```python
from build123d import *

# Parameters (mm, degrees)
SKETCH_1_R          = 40
EXTRUDE_1_DEPTH     = 50
CUT_EXTRUDE_1_DEPTH = 30
CUT_EXTRUDE_2_DEPTH = 76.498344353


with BuildPart() as part:
    # Sketch 1 → Extrude 1 (new body)
    with BuildSketch(Plane(origin=(0, 0, 0), x_dir=(1, 0, 0), z_dir=(0, 1, 0))):
        with Locations(Location((0, 0, 0), (0, 0, 270))):
            Circle(SKETCH_1_R)
    extrude(amount=EXTRUDE_1_DEPTH)

    # Sketch 2 → Cut-Extrude 1 (cut)
    with BuildSketch(Plane.XZ):
        with BuildLine():
            Line((18.540496218, 7.5), (25, 7.5))
            Line((25, 7.5), (25, -7.5))
            Line((25, -7.5), (18.540496218, -7.5))
            ThreePointArc((18.540496218, -7.5), (-20, 0), (18.540496218, 7.5))
        make_face()
    extrude(amount=-CUT_EXTRUDE_1_DEPTH, mode=Mode.SUBTRACT)

    # Sketch 4 → Cut-Extrude 2 (cut, through all)
    with BuildSketch(Plane.XZ):
        with BuildLine():
            Line((40, -2.5), (30, -2.5))
            ThreePointArc((30, -2.5), (27.5, 0), (30, 2.5))
            Line((30, 2.5), (40, 2.5))
            ThreePointArc((40, 2.5), (42.5, 0), (40, -2.5))
        make_face()
    extrude(amount=-CUT_EXTRUDE_2_DEPTH, mode=Mode.SUBTRACT)


solid = part.part
```
The model under review builds one solid part; all positions refer to its coordinate system, in mm. A direction names the side the tool comes from. Round coordinates to 2 decimals unless told otherwise and drop trailing zeros. Write each loop counter-clockwise with the first axis right and the second up, starting at its lowest first coordinate (ties: lowest second). Pieces come first, ordered by that corner, then holes. Notation, with made-up numbers: (67.25, -9.75) -> (111.25, -9.75) arc R12 ccw to (111.25, -1.75) -> close; hole circle Ø7 at (5.5, 19.5). An arc over 180 degrees is marked (long way). Use CSV: the item, a comma, the result in double quotes.
Q1. Consider section A-A (y = 22.5). Give the boundary of the cut face in (x, z).
Checks:
outline,"(30, -2.5) arc R2.5 cw to (30, 2.5) -> (39.92, 2.5) arc R40 ccw (long way) to (39.92, -2.5) -> close; hole (18.54, -7.5) -> (25, -7.5) -> (25, 7.5) -> (18.54, 7.5) arc R20 ccw (long way) to start"
Q2. Consider section B-B (z = 0). Give the boundary of the cut face in (x, y), then the cut area to 4 significant figures.
Checks:
outline,"(-40, 0) -> (-20, 0) -> (-20, 30) -> (25, 30) -> (25, 0) -> (27.5, 0) -> (27.5, 50) -> (-40, 50) -> close"
area,"2,025 mm²"
Q3. Mouldability with a two-part tool opening along Z and no side actions: class faces 4 (the flat face through (25, 15, 0)), 5 (the flat face through (-8.36, 0, -18.34)), 6 (the cylindrical face through (27.5, 24.6, -0.1)) as released by +Z, released by -Z, zero draft, split by the parting line, or undercut.
Checks:
face 4,"undercut"
face 5,"zero draft"
face 6,"undercut"
Q4. For pin 1 Ø3 at (y, z) = (7.5, -30.5) entering from +X; pin 2 Ø2 at (x, y) = (-5, 37.5) entering from +Z; pin 3 Ø11 at (x, y) = (33.5, 25.5) entering from +Z; pin 4 Ø4 at (x, z) = (32, -28) entering from -Y, all flat-tipped, find the tip position at first contact; note any pin that passes through.
Checks:
pin 1,"x = 27.55"
pin 2,"z = 39.8"
pin 3,"z = 28.57"
pin 4,"through"
Q5. Consider section C-C (x = -14.5). Give the boundary of the cut face in (y, z), then the cut area to 3 significant figures.
Checks:
outline,"(0, -37.28) -> (50, -37.28) -> (50, 37.28) -> (0, 37.28) -> (0, 13.77) -> (30, 13.77) -> (30, -13.77) -> (0, -13.77) -> close"
area,"2,900 mm²"
Q6. Consider section D-D (y = 39.5). Give the boundary of the cut face in (x, z), then the cut area to 3 significant figures.
Checks:
outline,"(30, -2.5) arc R2.5 cw to (30, 2.5) -> (39.92, 2.5) arc R40 ccw (long way) to (39.92, -2.5) -> close"
area,"4,970 mm²"
Q7. To check wall thickness, follow probe 1 along X at (y, z) = (17.5, 0); probe 2 along Y at (x, z) = (10, -3.5); probe 3 along Z at (x, y) = (0, 22.25). State the ranges of each line that lie inside material, in increasing order. Write a range as [from, to].
Checks:
probe 1,"[-40, -20], [25, 27.5]"
probe 2,"[30, 50]"
probe 3,"[-40, -20], [20, 40]"
Q8. For faces 1 (the flat face through (35, 25, 2.5)), 2 (the flat face through (1, 50, -1)), 3 (the flat face through (22, 15, -7.5)), list the 3-axis set-ups (+Z, -Z, +X, -X, +Y, -Y) from which the entire face can be reached by the end or side of a thin tool; tool diameter is ignored.
Checks:
face 1,"+X, +Y, -Y"
face 2,"+Z, -Z, +X, -X, +Y"
face 3,"-Y"
